Source: CAD feature listing. Evaluate the final solid. Frame: model axes, mm. Coordinates: 2 decimals unless noted, no trailing zeros. Write each loop counter-clockwise with the first axis right and the second up, starting at its lowest first coordinate (ties: lowest second). Pieces come first, ordered by that corner, then holes. Notation, with made-up numbers: M 86,46 L 138,46 A24 cw 138,78 Z; hole C 5,-17 d1. An arc over 180 degrees is marked long. One line per item, written item: value. Start each with the question number.
Item 1: Pin query (flat end, axial travel): P1, Ø4, axis at x = 40, y = 0, coming from the +Z side; P2, Ø1, axis at x = -9.5, z = 1, coming from the -Y side. Return the tip coordinate at first contact, or that it passes through.
Item 2: Cut plane B-B, the plane z = 2.95. Output: boundary loops of the cut face in (x, y).
Item 3: Cut plane D-D, the plane y = 0. Output: boundary loops of the cut face in (x, z).
Item 4: Cut plane A-A, the plane x = 0. Output: boundary loops of the cut face in (y, z).
Item 5: Ray query, L1, parallel to Z at x = 11.5, y = 10; L2, parallel to Y at x = 0, z = 0.9; L3, parallel to Y at x = 40, z = 0.7. Return the intervals inside material, ascending. Write a range as from..to.
Item 6: Cut plane C-C, the plane y = 28.4. Output: boundary loops of the cut face in (x, z).
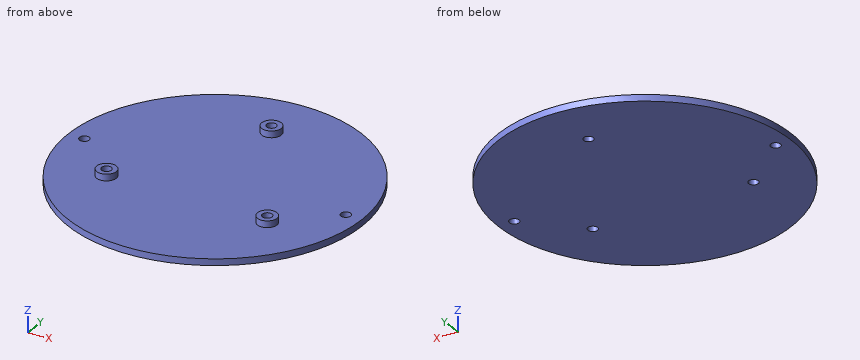
```python
from build123d import *

# Parameters (mm, degrees)
SKETCH_R     = 45
SKETCH_R_2   = 1.5
PAD_DEPTH    = 2
SKETCH001_R  = 3
PAD001_DEPTH = 2
SKETCH002_R  = 1.5
POCKET_DEPTH = 5


with BuildPart() as part:
    # Sketch → Pad (new body)
    with BuildSketch(Plane.XY):
        Circle(SKETCH_R)
        with Locations((-40, 0)):
            Circle(SKETCH_R_2, mode=Mode.SUBTRACT)
        with Locations((40, 0)):
            Circle(SKETCH_R_2, mode=Mode.SUBTRACT)
    extrude(amount=PAD_DEPTH)

    # Sketch001 (on Face5 of Pad) → Pad001 (join)
    with BuildSketch(Plane.XY.offset(2)):
        with Locations((-24.595121, -14.2)):
            Circle(SKETCH001_R)
        with Locations((0, 28.4)):
            Circle(SKETCH001_R)
        with Locations((24.595121, -14.2)):
            Circle(SKETCH001_R)
    extrude(amount=PAD001_DEPTH)

    # Sketch002 (on Face9 of Pad001) → Pocket (cut)
    with BuildSketch(Plane.XY.offset(4)):
        with Locations((-24.595121, -14.2)):
            Circle(SKETCH002_R)
        with Locations((0, 28.4)):
            Circle(SKETCH002_R)
        with Locations((24.595121, -14.2)):
            Circle(SKETCH002_R)
    extrude(amount=-POCKET_DEPTH, mode=Mode.SUBTRACT)


solid = part.part
```
From the geometry:
1. P1: stops at z = 2
1. P2: stops at y = -44.09
2. outline: C -24.6,-14.2 d6; C 0,28.4 d6; C 24.6,-14.2 d6; hole C -24.6,-14.2 d3; hole C 0,28.4 d3; hole C 24.6,-14.2 d3
3. outline: M -45,0 L -41.5,0 L -41.5,2 L -45,2 Z; M -38.5,0 L 38.5,0 L 38.5,2 L -38.5,2 Z; M 41.5,0 L 45,0 L 45,2 L 41.5,2 Z
4. outline: M -45,0 L 26.9,0 L 26.9,4 L 25.4,4 L 25.4,2 L -45,2 Z; M 29.9,0 L 45,0 L 45,2 L 31.4,2 L 31.4,4 L 29.9,4 Z
5. L1: z = 0..2
5. L2: y = -45..26.9, 29.9..45
5. L3: y = -20.62..-1.5, 1.5..20.62
6. outline: M -34.91,0 L -1.5,0 L -1.5,4 L -3,4 L -3,2 L -34.91,2 Z; M 1.5,0 L 34.91,0 L 34.91,2 L 3,2 L 3,4 L 1.5,4 Z
